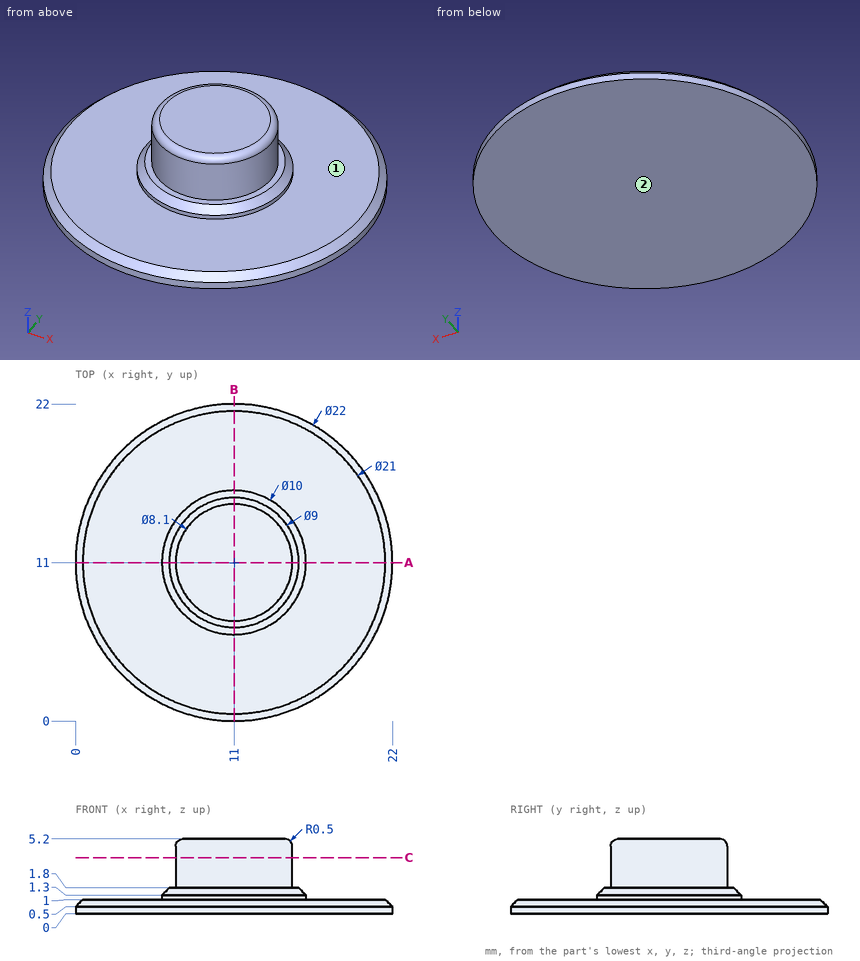
Study the drawing (mm; zero at the part's minimum x, y, z) and answer. A direction names the side the tool comes from. Coordinates: 2 decimals unless noted, no trailing zeros. Write each loop counter-clockwise with the first axis right and the second up, starting at its lowest first coordinate (ties: lowest second). Pieces come first, ordered by that corner, then holes. Notation, with made-up numbers: (19, -8.5) -> (46, -8.5) arc R33 cw to (46, 21.5) -> close; hole circle Ø11 at (-5.5, 9.25). An arc over 180 degrees is marked (long way). Write each question's results on one line, items separated by ' | '. Start each with the question number.
1) A tool of negligible diameter and unlimited length cuts with its end or side. For the marked faces 1 and 2, from which of +Z, -Z, +X, -X, +Y, -Y can it reach the whole face along a straight path? Write none if from no direction.
2) A cutting plane is placed at A-A (y = 11). Determine the outline of the cut face in (x, z).
3) Flat-ended cylindrical pins translate along their axes: pin 1 Ø3 at (y, z) = (13, 3) entering from -X; pin 2 Ø3 at (y, z) = (9.5, 2) entering from -X; pin 3 Ø1 at (x, z) = (6, 4.5) entering from -Y; pin 4 Ø3 at (x, z) = (10.5, 3) entering from -Y. Find the tip coordinate at first contact, or state that the pin passes through.
4) A cutting plane is placed at C-C (z = 3.9). Determine the outline of the cut face in (x, y), then the cut area to 3 significant figures.
5) Straight lines are drawn through the part: probe 1 along Y at (x, z) = (11, 2.45); probe 2 along Z at (x, y) = (9.5, 2.5); probe 3 along Z at (x, y) = (7.75, 14). For each, find the intervals that lie inside material, in ascending order.
Values follow:
1) face 1: +Z | face 2: -Z, +X, -X, +Y, -Y
2) outline: (0, 0) -> (22, 0) -> (22, 0.5) -> (21.5, 1) -> (16, 1) -> (16, 1.3) -> (15.5, 1.8) -> (15.05, 1.8) -> (15.05, 4.7) arc R0.5 ccw to (14.55, 5.2) -> (7.45, 5.2) arc R0.5 ccw to (6.95, 4.7) -> (6.95, 1.8) -> (6.5, 1.8) -> (6, 1.3) -> (6, 1) -> (0.5, 1) -> (0, 0.5) -> close
3) pin 1: x = 6.53 | pin 2: x = 0.09 | pin 3: through | pin 4: y = 6.22
4) outline: circle Ø8.1 at (11, 11) | area: 51.5 mm²
5) probe 1: 6.95 to 15.05 | probe 2: 0 to 1 | probe 3: 0 to 1.8
